For this review, take the finished solid that the model builds, in its own axes (mm). A direction names the side the tool comes from. Give positions to 0.01 mm unless a question says otherwise; leave off trailing zeros. Write each loop counter-clockwise with the first axis right and the second up, starting at its lowest first coordinate (ties: lowest second). Pieces come first, ordered by that corner, then holes. Notation, with made-up numbers: (87.25, -7.75) -> (125.25, -7.75) arc R12 cw to (125.25, 1.25) -> close; hole circle Ø1 at (86.5, 43.5). An arc over 180 degrees is marked (long way). Return JSON: item names as keys, results as strings.
from build123d import *

# Parameters (mm, degrees)
FRAME_AND_BENCH_INTERFACE_START = -1
PROFILE_1_R                     = 20
PROFILE_1_R_2                   = 3.25
PROFILE_1_R_3                   = 1.65
PROFILE_1_R_4                   = 2.65
FRAME_AND_BENCH_INTERFACE_DEPTH = 8
RECESS_STATOR_SCREW_HEADS_START = 3.1
PROFILE_2_R                     = 3.05
RECESS_STATOR_SCREW_HEADS_DEPTH = 4
REAR_CAPTIVE_NUT_B_START        = -1.01
REAR_CAPTIVE_NUT_B_DEPTH        = 4.51


with BuildPart() as part:
    # Profile_1 → Frame_and_bench_interface (new body)
    with BuildSketch(Plane.XY.offset(FRAME_AND_BENCH_INTERFACE_START)):
        Polygon((-58.865496963, 13.365632254), (-58.865496963, -63.365632254), (-57.820287286, -65.888991631), (-55.888991631, -67.820287286), (-53.365632254, -68.865496963), (-2.731264508, -75.730993926), (2.731264508, -75.730993926), (7.777983262, -73.640574572), (11.640574572, -69.777983262), (13.730993926, -64.731264508), (32.365914253, -6.437980627), (32.365914253, 6.437980627), (27.438497206, 18.33381769), (18.33381769, 27.438497206), (6.437980627, 32.365914253), (-6.437980627, 32.365914253), (-53.365632254, 18.865496963), (-55.888991631, 17.820287286), (-57.820287286, 15.888991631), align=None)
        Circle(PROFILE_1_R, mode=Mode.SUBTRACT)
        with Locations((0, -62)):
            Circle(PROFILE_1_R_2, mode=Mode.SUBTRACT)
        with Locations((21.650635095, 12.5)):
            Circle(PROFILE_1_R_3, mode=Mode.SUBTRACT)
        with Locations((0, 25)):
            Circle(PROFILE_1_R_3, mode=Mode.SUBTRACT)
        with Locations((-21.650635095, 12.5)):
            Circle(PROFILE_1_R_3, mode=Mode.SUBTRACT)
        with Locations((-21.650635095, -12.5)):
            Circle(PROFILE_1_R_3, mode=Mode.SUBTRACT)
        with Locations((0, -25)):
            Circle(PROFILE_1_R_3, mode=Mode.SUBTRACT)
        with Locations((21.650635095, -12.5)):
            Circle(PROFILE_1_R_3, mode=Mode.SUBTRACT)
        with Locations((-52, 12)):
            Circle(PROFILE_1_R_4, mode=Mode.SUBTRACT)
        with Locations((-37, 12)):
            Circle(PROFILE_1_R_4, mode=Mode.SUBTRACT)
        with Locations((-52, -62)):
            Circle(PROFILE_1_R_4, mode=Mode.SUBTRACT)
        with Locations((-37, -62)):
            Circle(PROFILE_1_R_4, mode=Mode.SUBTRACT)
    extrude(amount=FRAME_AND_BENCH_INTERFACE_DEPTH)

    # Profile_2 → Recess_stator_screw_heads (cut)
    with BuildSketch(Plane.XY.offset(RECESS_STATOR_SCREW_HEADS_START)):
        with Locations((21.650635095, 12.5)):
            Circle(PROFILE_2_R)
        with Locations((0, 25)):
            Circle(PROFILE_2_R)
        with Locations((-21.650635095, 12.5)):
            Circle(PROFILE_2_R)
        with Locations((-21.650635095, -12.5)):
            Circle(PROFILE_2_R)
        with Locations((0, -25)):
            Circle(PROFILE_2_R)
        with Locations((21.650635095, -12.5)):
            Circle(PROFILE_2_R)
    extrude(amount=RECESS_STATOR_SCREW_HEADS_DEPTH, mode=Mode.SUBTRACT)

    # Profile_3 → Rear_captive_nut_B (cut)
    with BuildSketch(Plane.XY.offset(REAR_CAPTIVE_NUT_B_START)):
        Polygon((5.175, -59.012212357), (0, -56.024424714), (-5.175, -59.012212357), (-5.175, -64.987787643), (0, -67.975575286), (5.175, -64.987787643), align=None)
    extrude(amount=REAR_CAPTIVE_NUT_B_DEPTH, mode=Mode.SUBTRACT)


solid = part.part
1. For pin 1 (1.5 mm diameter, centred on x = -37.5, z = 1.5, fed in from -Y); pin 2 (10 mm diameter, centred on x = 0, y = 25, fed in from +Z); pin 3 (2 mm diameter, centred on x = -41, z = 1, fed in from -Y); pin 4 (1.8 mm diameter, centred on x = -1, y = -24, fed in from +Z), all flat-tipped, find the tip position at first contact; note any pin that passes through.
Results found:
{"pin 1": "stops at y = -71.12", "pin 2": "stops at z = 7", "pin 3": "stops at y = -70.68", "pin 4": "stops at z = 3.1"}
2. To check wall thickness, follow probe 1 along Y at (x, z) = (3, 2.25); probe 2 along X at (y, z) = (12.5, 5.7); probe 3 along X at (y, z) = (-12.5, 3.95). State the ranges of each line that lie inside material, in increasing order.
Results found:
{"probe 1": "y = -75.62 to -66.24, -57.76 to -19.77, 19.77 to 32.37", "probe 2": "x = -58.87 to -54.6, -49.4 to -39.6, -34.4 to -24.7, -18.6 to -15.61, 15.61 to 18.6, 24.7 to 29.85", "probe 3": "x = -58.87 to -24.7, -18.6 to -15.61, 15.61 to 18.6, 24.7 to 30.43"}
3. For faces 1 (the flat face through (-2.624, -66.461, 1.218)), 2 (the flat face through (22.92, -35.99, 2.94)), 3 (the cylindrical face through (-2.25, -22.94, 5.02)), list the 3-axis set-ups (+Z, -Z, +X, -X, +Y, -Y) from which the entire face can be reached by the end or side of a thin tool; tool diameter is ignored.
Results found:
{"face 1": "-Z", "face 2": "+Z, -Z, +X, -Y", "face 3": "+Z"}
4. The part is to be moulded in two halves that separate along X. For faces 4 (the flat face through (5.22, -74.7, 2.94)), 5 (the cylindrical face through (-49.55, 10.99, 2.94)), 6 (the flat face through (-14, -21, -1)), say which applies: +X half, -X half, draft (parallel to the pull), parting line (faces both ways), or undercut.
Results found:
{"face 4": "+X half", "face 5": "undercut", "face 6": "draft"}
5. Add section A-A, the plane z = 5.25. Count the separate pieces of the cut face and the enclosed holes in it, plus the area to 3 significant figures.
Results found:
{"separate pieces": "1", "enclosed holes": "12", "area": "6,690 mm²"}
6. Add section B-B, the plane y = -25. State the section outline as (x, z) points.
Results found:
{"outline": "(-58.87, -1) -> (-1.65, -1) -> (-1.65, 3.1) -> (-3.05, 3.1) -> (-3.05, 7) -> (-58.87, 7) -> close; (1.65, -1) -> (26.43, -1) -> (26.43, 7) -> (3.05, 7) -> (3.05, 3.1) -> (1.65, 3.1) -> close"}
7. Add section D-D, the plane x = -37. State the section outline as (y, z) points, plus the area to 3 significant figures.
Results found:
{"outline": "(-71.08, -1) -> (-64.65, -1) -> (-64.65, 7) -> (-71.08, 7) -> close; (-59.35, -1) -> (9.35, -1) -> (9.35, 7) -> (-59.35, 7) -> close; (14.65, -1) -> (23.57, -1) -> (23.57, 7) -> (14.65, 7) -> close", "area": "672 mm²"}
